```python
from build123d import *

# Parameters (mm, degrees)
F0_W     = 28
F0_H     = 59
F1_DEPTH = 5.5
F2_W     = 5
F2_H     = 3
F3_DEPTH = 1.5
F4_W     = 4
F4_H     = 2
F5_DEPTH = 4
F6_D     = 2.2
F6_DEPTH = 5


with BuildPart() as f1:
    # F0 (on Top) → F1 (new body)
    with BuildSketch(Plane.XY):
        Rectangle(F0_W, F0_H)
    extrude(amount=F1_DEPTH)

    # F2 (on Top) → F3 (join)
    with BuildSketch(Plane.XY):
        with Locations((0, -31)):
            Rectangle(F2_W, F2_H)
    extrude(amount=F3_DEPTH)

    # F4 (on face) → F5 (join)
    with BuildSketch(Plane.XY.offset(5.5)):
        with Locations((0, 30.5)):
            Rectangle(F4_W, F4_H)
        with BuildLine():
            ThreePointArc((2, 31.5), (0, 33.5), (-2, 31.5))
            Line((-2, 31.5), (2, 31.5))
        make_face()
    extrude(amount=-F5_DEPTH)

    # F6
    with Locations(Plane.XY.offset(5.5)):
        with Locations((0, 31.5)):
            Hole(F6_D / 2, depth=F6_DEPTH)


solid = f1.part
```
Geometry check sheet. Reference: the model listing, model coordinates, mm. A direction names the side the tool comes from. Round coordinates to 2 decimals unless told otherwise and drop trailing zeros. Order: outer loops, then holes, each group sorted by start corner. A loop starts at its lowest first (then second) coordinate and runs counter-clockwise, first axis right, second up. Notation, with made-up numbers: (-37.75, 31) -> (12.25, 31) arc R12 cw to (12.25, 41) -> close; hole circle Ø10 at (29, 2.25). An arc over 180 degrees is marked (long way). Return JSON: item names as keys, results as strings. Group by question number.
Q1. Gauge pin test, flat ends, axial feed: pin 1 (1.5 mm diameter, centred on x = -1, y = -30.5, fed in from +Z); pin 2 (1.6 mm diameter, centred on y = 31, z = 4, fed in from -X); pin 3 (1.6 mm diameter, centred on x = 1, z = 2.5, fed in from +Y). Record the tip position at first contact, or that the pin passes through.
Q2. Tool access check on faces 4 (the flat face through (0, -31, 1.5)), 5 (the flat face through (-2, 30, 4)), 6 (the flat face through (0.9, 30.6, 1.5)). Record the directions out of +Z, -Z, +X, -X, +Y, -Y that give a thin tool (end or side, any length) a straight path to the whole face; none if there is none.
Q3. Section check C-C, the plane z = 0.6. Record the boundary of the cut face in (x, y), plus the area to 3 significant figures.
Q4. Section check B-B, the plane z = 4.4. Record the boundary of the cut face in (x, y).
Q5. Material ranges on probe 1 along Y at (x, z) = (0, 3.5); probe 2 along Y at (x, z) = (8.75, 1.05); probe 3 along Y at (x, z) = (-1.5, 2.6), recorded low to high. Write a range as from..to.
Q6. Section check A-A, the plane x = 0. Record the boundary of the cut face in (y, z).
Q7. Release check for a two-part mould opening along X. For faces 1 (the flat face through (2.5, -31, 1)), 2 (the cylindrical face through (-0.59, 32.43, 3.47)), 3 (the cylindrical face through (0, 33.5, 3.5)) record: released by +X, released by -X, zero draft, split by the parting line, or undercut.
Q8. Section check D-D, the plane x = -12. Record the boundary of the cut face in (y, z), plus the area to 4 significant figures.
Numbers:
{
 "1": {"pin 1": "z = 1.5", "pin 2": "x = -2", "pin 3": "y = 33.49"},
 "2": {"face 4": "+Z, +X, -X, -Y", "face 5": "+Z, -Z, -X, +Y", "face 6": "-Z, +X, -X, +Y"},
 "3": {"outline": "(-14, -29.5) -> (-2.5, -29.5) -> (-2.5, -32.5) -> (2.5, -32.5) -> (2.5, -29.5) -> (14, -29.5) -> (14, 29.5) -> (-14, 29.5) -> close", "area": "1,670 mm^2"},
 "4": {"outline": "(-14, -29.5) -> (14, -29.5) -> (14, 29.5) -> (2, 29.5) -> (2, 31.5) arc R2 ccw to (-2, 31.5) -> (-2, 29.5) -> (-14, 29.5) -> close; hole circle Ø2.2 at (0, 31.5)"},
 "5": {"probe 1": "-29.5..30.4, 32.6..33.5", "probe 2": "-29.5..29.5", "probe 3": "-29.5..32.82"},
 "6": {"outline": "(-32.5, 0) -> (29.5, 0) -> (29.5, 1.5) -> (30.4, 1.5) -> (30.4, 5.5) -> (-29.5, 5.5) -> (-29.5, 1.5) -> (-32.5, 1.5) -> close; (32.6, 1.5) -> (33.5, 1.5) -> (33.5, 5.5) -> (32.6, 5.5) -> close"},
 "7": {"face 1": "released by +X", "face 2": "undercut", "face 3": "split by the parting line"},
 "8": {"outline": "(-29.5, 0) -> (29.5, 0) -> (29.5, 5.5) -> (-29.5, 5.5) -> close", "area": "324.5 mm^2"}
}
